Autodesk Inventor part; units mm, degrees
ref_plane "YZ Plane" through (0, 0, 0) normal (1, 0, 0) x (0, 1, 0)
ref_plane "XZ Plane" through (0, 0, 0) normal (0, 1, 0) x (-1, 0, 0)
ref_plane "XY Plane" through (0, 0, 0) normal (0, 0, 1) x (1, 0, 0)
sketch "スケッチ1" plane through (0, 0, 0) normal (0, 0, 1) x (1, 0, 0)
  line L0 (-15, 65) -> (15, 65)
  line L1 (15, 65) -> (15, 47.1)
  line L2 (15, -65) -> (-15, -65)
  line L3 (-15, -65) -> (-15, -47.1)
  line L4 (-15, 65) -> (15, -65) construction
  line L5 (15, 65) -> (-15, -65) construction
  line L6 (-15, 45) -> (-20, 45)
  line L7 (-20, 45) -> (-20, 45)
  line L8 (-20, 15) -> (-15, 15)
  line L9 (-20, 15) -> (-20, 45)
  line L10 (-15, -15) -> (-20, -15)
  line L11 (-20, -15) -> (-20, -45)
  line L12 (-20, -45) -> (-15, -45)
  arc A0 (-15, 45) -> (-15, 47.1) centre (-15, 46.05) ccw
  arc A1 (-15, 12.9) -> (-15, 15) centre (-15, 13.95) ccw
  arc A2 (-15, -15) -> (-15, -12.9) centre (-15, -13.95) ccw
  arc A3 (-15, -47.1) -> (-15, -45) centre (-15, -46.05) ccw
  line L13 (-15, 47.1) -> (-15, 65)
  line L14 (-15, 12.9) -> (-15, 47.1) construction
  line L15 (-15, -12.9) -> (-15, 12.9)
  line L16 (-15, -47.1) -> (-15, -45) construction
  line L17 (0, 65) -> (0, -65) construction
  line L18 (15, 45) -> (20, 45)
  line L19 (20, 15) -> (15, 15)
  line L20 (20, 15) -> (20, 45)
  line L21 (15, -15) -> (20, -15)
  line L22 (20, -15) -> (20, -45)
  line L23 (20, -45) -> (15, -45)
  arc A4 (15, 47.1) -> (15, 45) centre (15, 46.05) ccw
  arc A5 (15, 15) -> (15, 12.9) centre (15, 13.95) ccw
  arc A6 (15, -12.9) -> (15, -15) centre (15, -13.95) ccw
  arc A7 (15, -45) -> (15, -47.1) centre (15, -46.05) ccw
  line L24 (15, 47.1) -> (15, 12.9) construction
  line L25 (15, 12.9) -> (15, -12.9)
  line L26 (15, -47.1) -> (15, -65)
  line L27 (15, -12.9) -> (15, -15) construction
  circle A8 centre (-17.5, 40) radius 1.55
  circle A9 centre (-17.5, 20) radius 1.55
  circle A10 centre (17.5, 20) radius 1.55
  circle A11 centre (17.5, 40) radius 1.55
  line L28 (-15, -15) -> (-15, -12.9) construction
  line L29 (-15, -45) -> (-15, -15)
  line L30 (15, -15) -> (15, -45)
  line L31 (15, -45) -> (15, -47.1) construction
  point P0 (0, 0)
  dimension "d8" = 30
  dimension "d9" = 130
  dimension "d10" = 20
  dimension "d11" = 30
  dimension "d12" = 30
  dimension "d13" = 30
  dimension "d16" = 1.05
  dimension "d17" = 1.05
  dimension "d18" = 1.05
  dimension "d19" = 1.05
  dimension "d20" = 5
  dimension "d23" = 20
  dimension "d24" = 5
  dimension "d25" = 5
  dimension "d28" = 2.5
  dimension "d29" = 2.5
  dimension "d33" = 3.1
  dimension "d38" = 3.1
  dimension "d39" = 20
extrude "押し出し1" add sketch "スケッチ1" along normal blind 2.5
extrude "押し出し2" add sketch "スケッチ1" along normal blind 5 contours L0 L1 A4 L18 L20 L19 A5 L25 A6 L30 A7 L26 L2 L3 A3 L29 A2 L15 A1 L8 L9 L6 A0 L13
chamfer "面取り1" distance 0.5 angle 45 4 edges at (20, -15, 1.25) (20, -45, 1.25) (-20, -15, 1.25) (-20, -45, 1.25)
equation "\"d10\" = -0.5 * d12 + 0.5 * d9 - d11"
equation "\"d13\" = d11"
equation "\"d17\" = d16"
equation "\"d18\" = d17"
equation "\"d19\" = d18"
equation "\"d25\" = d24"
equation "\"d28\" = 0.5 * d20"
equation "\"d29\" = d28"
equation "\"d33\" = d38"
properties part number "Cockpit_lower_bottom_frame" material "アセタール樹脂、黒"
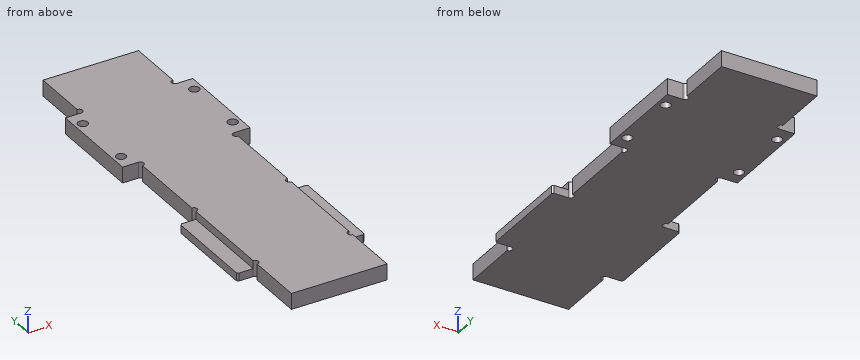
Input: part model. Units: mm. Frame: model coordinates. Coordinates: 2 decimals unless noted, no trailing zeros. Order: outer loops, then holes, each group sorted by start corner. A loop starts at its lowest first (then second) coordinate and runs counter-clockwise, first axis right, second up. Notation, with made-up numbers: M 27,43 L 78,43 A12 cw 78,47 Z; hole C 26.25,60 d3. An arc over 180 degrees is marked long. One line per question, with ' | ' between items.
Item 1: Section B-B (x = 17.5). Output: boundary loops of the cut face in (y, z), then the cut area to 3 significant figures.
Geometry results:
outline: M -45,0 L -15,0 L -15,2.5 L -45,2.5 Z; M 15,0 L 18.45,0 L 18.45,5 L 15,5 Z; M 21.55,0 L 38.45,0 L 38.45,5 L 21.55,5 Z; M 41.55,0 L 45,0 L 45,5 L 41.55,5 Z | area: 194 mm^2
Item 2: Section A-A (y = 40). Output: boundary loops of the cut face in (x, z).
Geometry results:
outline: M -20,0 L -19.05,0 L -19.05,5 L -20,5 Z; M -15.95,0 L 15.95,0 L 15.95,5 L -15.95,5 Z; M 19.05,0 L 20,0 L 20,5 L 19.05,5 Z
Item 3: Ray query, line 1 along Y through (x, z) = (17.5, 3.6); line 2 along Y through (x, z) = (-17.5, 1.4); line 3 along Z through (x, y) = (15.5, -43.5). Return the intervals inside material, ascending.
Geometry results:
line 1: y = 15 to 18.45, 21.55 to 38.45, 41.55 to 45 | line 2: y = -45 to -15, 15 to 18.45, 21.55 to 38.45, 41.55 to 45 | line 3: z = 0 to 2.5
Item 4: Pin query (flat end, axial travel): pin 1 (3 mm diameter, centred on y = 50, z = 3.5, fed in from +X); pin 2 (2 mm diameter, centred on x = 16.5, z = 1, fed in from +Y); pin 3 (1.2 mm diameter, centred on x = -16, z = 1.5, fed in from -Y); pin 4 (2.5 mm diameter, centred on x = 17.5, y = 20, fed in from -Z). Return the tip coordinate at first contact, or that it passes through.
Geometry results:
pin 1: stops at x = 15 | pin 2: stops at y = 45 | pin 3: stops at y = -45 | pin 4: passes through
Item 5: Section C-C (z = 1.45). Give the number of separate pieces and of enclosed holes in the cut face, then the cut area to 3 significant figures.
Geometry results:
separate pieces: 1 | enclosed holes: 4 | area: 4,460 mm^2
